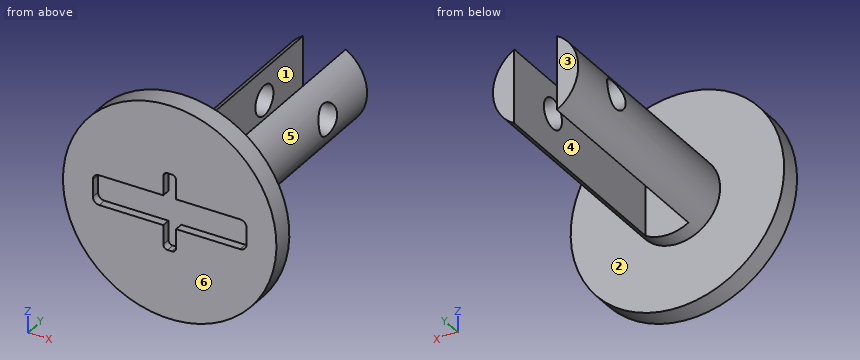
from build123d import *

# Parameters (mm, degrees)
SKETCH1_R           = 10
BOSS_EXTRUDE1_DEPTH = 60
SKETCH1_5_R         = 25
SKETCH1_5_R_2       = 10
BOSS_EXTRUDE3_DEPTH = 5
SKETCH6_W           = 10
SKETCH6_H           = 20
CUT_EXTRUDE2_DEPTH  = 51
CUT_EXTRUDE3_START  = -10.0000001
CUT_EXTRUDE3_DEPTH  = 20.000000175
SKETCH8_W           = 1.5
SKETCH8_H           = 5.5075
SKETCH8_H_2         = 3.4925
SKETCH8_W_2         = 16.5
CUT_EXTRUDE4_DEPTH  = 2
FILLET2_R           = 1.5
FILLET3_R           = 1


# Read off the part's stored shape, not the designer's step: Cut-Extrude3
with BuildPart() as part:
    # Sketch1 → Boss-Extrude1 (new body)
    with BuildSketch(Plane(origin=(0, 0, 0), x_dir=(1, 0, 0), z_dir=(0, 1, 0))):
        with Locations(Location((0, 0, 0), (0, 0, 270))):
            Circle(SKETCH1_R)
    extrude(amount=BOSS_EXTRUDE1_DEPTH)

    # Sketch1<5> → Boss-Extrude3 (add)
    with BuildSketch(Plane(origin=(0, 0, 0), x_dir=(1, 0, 0), z_dir=(0, 1, 0))):
        with Locations(Location((0, 0, 0), (0, 0, 270))):
            Circle(SKETCH1_5_R)
        with Locations(Location((0, 0, 0), (0, 0, 270))):
            Circle(SKETCH1_5_R_2, mode=Mode.SUBTRACT)
    extrude(amount=BOSS_EXTRUDE3_DEPTH)

    # Sketch6 → Cut-Extrude2 (cut)
    with BuildSketch(Plane(origin=(0, 60, 0), x_dir=(1, 0, 0), z_dir=(0, 1, 0))):
        Rectangle(SKETCH6_W, SKETCH6_H)
    extrude(amount=-CUT_EXTRUDE2_DEPTH, mode=Mode.SUBTRACT)

    # Cut-Extrude3 outline → Cut-Extrude3 (cut)
    with BuildSketch(Plane(origin=(0, 0, 0), x_dir=(0, 0, -1), z_dir=(1, 0, 0)).offset(CUT_EXTRUDE3_START)):
        with BuildLine():
            add(Edge.make_bspline(
                [(-4.839745962, 45), (-4.839745962, 44.061427817), (-4.450746498, 43.166577946), (-3.199248606, 41.904517699), (-2.320388043, 41.517275442), (-0.486539081, 41.483884635), (0.452391521, 41.853887629), (1.774975913, 43.153845226), (2.16014876, 44.075410749), (2.16035927, 45.923792027), (1.777989156, 46.84346553), (0.448336969, 48.149824894), (-0.485336071, 48.515908682), (-2.319848282, 48.482962757), (-3.200529308, 48.095220586), (-4.45348427, 46.829628074), (-4.839745962, 45.938572183), (-4.839745962, 45)],
                knots=[0, 0, 0, 0, 0.125, 0.125, 0.25, 0.25, 0.375, 0.375, 0.5, 0.5, 0.625, 0.625, 0.75, 0.75, 0.875, 0.875, 1, 1, 1, 1], degree=3))
        make_face()
    extrude(amount=CUT_EXTRUDE3_DEPTH, mode=Mode.SUBTRACT)

    # Sketch8 → Cut-Extrude4 (cut)
    with BuildSketch(Plane.XZ):
        with Locations((-0.75, -6.24625)):
            Rectangle(SKETCH8_W, SKETCH8_H)
        with Locations((0.75, -6.24625)):
            Rectangle(SKETCH8_W, SKETCH8_H)
        with Locations((0.75, -1.74625)):
            Rectangle(SKETCH8_W, SKETCH8_H_2)
        with Locations((-0.75, -1.74625)):
            Rectangle(SKETCH8_W, SKETCH8_H_2)
        with Locations((9.75, -1.74625)):
            Rectangle(SKETCH8_W_2, SKETCH8_H_2)
        with Locations((9.75, 1.74625)):
            Rectangle(SKETCH8_W_2, SKETCH8_H_2)
        with Locations((0.75, 1.74625)):
            Rectangle(SKETCH8_W, SKETCH8_H_2)
        with Locations((-0.75, 1.74625)):
            Rectangle(SKETCH8_W, SKETCH8_H_2)
        with Locations((0.75, 6.24625)):
            Rectangle(SKETCH8_W, SKETCH8_H)
        with Locations((-0.75, 6.24625)):
            Rectangle(SKETCH8_W, SKETCH8_H)
        with Locations((-9.75, 1.74625)):
            Rectangle(SKETCH8_W_2, SKETCH8_H_2)
        with Locations((-9.75, -1.74625)):
            Rectangle(SKETCH8_W_2, SKETCH8_H_2)
    extrude(amount=-CUT_EXTRUDE4_DEPTH, mode=Mode.SUBTRACT)

    # Fillet2
    fillet2_edges = [part.edges().sort_by_distance(p)[0] for p in [
        (18, 1, 3.4925),
        (18, 1, -3.4925),
        (-18, 1, -3.4925),
        (-18, 1, 3.4925),
    ]]
    fillet(fillet2_edges, radius=FILLET2_R)

    # Fillet3
    fillet3_edges = [part.edges().sort_by_distance(p)[0] for p in [
        (1.5, 1, -9),
        (-1.5, 1, -9),
        (-1.5, 1, 9),
        (1.5, 1, 9),
    ]]
    fillet(fillet3_edges, radius=FILLET3_R)


solid = part.part
Could you check a few things on this model? Use its own coordinates, in mm. Face numbers are marked on the shaded views. A direction names the side the tool comes from. Give positions to 0.01 mm unless a question says otherwise; leave off trailing zeros. Loops run counter-clockwise (first coordinate to the right, second up) from the corner with the lowest first, then second, coordinate; pieces in that order, holes last. Notation, with made-up numbers: (53, -33) -> (109, -33) arc R29 ccw to (109, -13) -> close; hole circle Ø5 at (64.25, 31.5). An arc over 180 degrees is marked (long way). Answer as CSV lines item,"result". Start each with the question number.
(1) If we section it at D-D on z = 15: Write out the boundary of the cut face in (x, y), then the cut area to 3 significant figures.
(2) If we section it at C-C on z = 0: Count the separate pieces of the cut face and the enclosed holes in it, then the cut area to 3 significant figures.
(3) Which directions (+Z, -Z, +X, -X, +Y, -Y) give clear straight access to the entire face, cutting with the end or side of a thin tool? Please do the marked faces 1, 2 and 3.
(4) If we section it at B-B on x = -13.5: Write out the boundary of the cut face in (y, z).
(5) I need wall thicknesses on probe 1 along X at (y, z) = (25, 0); probe 2 along Y at (x, z) = (14, 11.5); probe 3 along X at (y, z) = (54, 5.5). Which ranges of each line are inside material? Lowest first, please.
(6) We'd pull the mould along X, two halves only. Please class the marked faces 4, 5 and 6: released by +X, released by -X, zero draft, split by the parting line, or undercut.
(7) I'm going to push flat-ended pins straight in: pin 1 Ø2 at (y, z) = (1.5, -4.5) entering from -X; pin 2 Ø2 at (y, z) = (1.5, 6) entering from +X; pin 3 Ø2 at (y, z) = (1.5, -5) entering from +X. Where does each tip first touch, or does it pass through?
(8) If we section it at A-A on y = 36: Write out the boundary of the cut face in (x, z), then the cut area to 3 significant figures.
Computed:
1,outline,"(-20, 0) -> (20, 0) -> (20, 5) -> (-20, 5) -> close"
1,area,"200 mm2"
2,separate pieces,"3"
2,enclosed holes,"0"
2,area,"703 mm2"
3,face 1,"+Z, -Z, +Y"
3,face 2,"+Y"
3,face 3,"+Z, -Z, +X, -X, +Y"
4,outline,"(0, -21.04) -> (5, -21.04) -> (5, 21.04) -> (0, 21.04) -> (0, 3.49) -> (2, 3.49) -> (2, -3.49) -> (0, -3.49) -> close"
5,probe 1,"x = -10 to -5, 5 to 10"
5,probe 2,"y = 0 to 5"
5,probe 3,"x = -8.35 to -5, 5 to 8.35"
6,face 4,"undercut"
6,face 5,"split by the parting line"
6,face 6,"zero draft"
7,pin 1,"stops at x = -24.75"
7,pin 2,"stops at x = 24.49"
7,pin 3,"stops at x = 24.68"
8,outline,"(-5, -8.66) -> (-5, 8.66) arc R10 ccw to start; (5, -8.66) arc R10 ccw to (5, 8.66) -> close"
8,area,"123 mm2"
